The listing builds one solid part. Answer for the finished solid, in the listing's coordinates (mm). Round coordinates to 2 decimals unless told otherwise and drop trailing zeros. Loops run counter-clockwise (first coordinate to the right, second up) from the corner with the lowest first, then second, coordinate; pieces in that order, holes last. Notation, with made-up numbers: M -38,-22.75 L 15,-22.75 A33 cw 15,6.25 Z; hole C 81.25,26.5 d9. An arc over 180 degrees is marked long. Put each result on its own line as item: value. Start each with the question number.
(1) Determine the mould class of faces 1 (the face through (-5, 0, 50)), 2 (the face through (-0.59, -4.46, -0.7)), 3 (the face through (-1.19, -5.37, 32.75)) for opening direction Y: released by +Y, released by -Y, zero draft, split by the parting line, or undercut.
(2) Section D-D, the plane z = -38 is taken. Determine the outline of the cut face in (x, y), then the cut area to 3 significant figures.
(3) Straight lines are drawn through the part: line 1 (Y direction, x = 0, z = 19); line 2 (Y direction, x = 0, z = 7); line 3 (X direction, y = -0.75, z = 23.5). For each, find the intervals that lie inside material, in ascending order.
(4) Section C-C, the plane z = 22.5 is taken. Determine the outline of the cut face in (x, y).
(5) Flat-ended cylindrical pins translate along their axes: P1, Ø5.5, axis at x = 1, y = 0.5, coming from the -Z side; P2, Ø2, axis at x = 1, z = 17.5, coming from the -Y side; P3, Ø4, axis at y = 3, z = 11.5, coming from the +X side; P4, Ø1, axis at y = 4.5, z = 7.5, coming from the -X side. Find the tip coordinate at first contact, or state that the pin passes through.
(6) Section A-A, the plane y = 0 is taken. Determine the outline of the cut face in (x, z), then the cut area to 3 significant figures.
```python
from build123d import *

# Parameters (mm, degrees)
F0_R     = 5
F1_DEPTH = 50
F3_R     = 4.5
F4_DEPTH = 100
F5_R     = 5.5
F5_R_2   = 5
F6_DEPTH = 35


with BuildPart() as f1:
    # F0 (on Top) → F1 (new body)
    with BuildSketch(Plane.XY):
        Circle(F0_R)
    extrude(amount=F1_DEPTH)

    # F2: F1 across face


with BuildPart() as f1_1:
    add(f1.part)
    add(f1.part.mirror(Plane(origin=(0, 0, 0), x_dir=(1, 0, 0), z_dir=(0, 0, -1))))

    # F3 (on face) → F4 (cut)
    with BuildSketch(Plane(origin=(0, 0, -50), x_dir=(1, 0, 0), z_dir=(0, 0, -1))):
        Circle(F3_R)
    extrude(amount=-F4_DEPTH, mode=Mode.SUBTRACT)

    # F5 (on face) → F6 (join)
    with BuildSketch(Plane.XY.offset(50)):
        Circle(F5_R)
        Circle(F5_R_2, mode=Mode.SUBTRACT)
    extrude(amount=-F6_DEPTH)


solid = f1_1.part
```
Recorded:
1. face 1: zero draft
1. face 2: undercut
1. face 3: split by the parting line
2. outline: C 0,0 d10; hole C 0,0 d9
2. area: 14.9 mm²
3. line 1: y = -5.5 to -4.5, 4.5 to 5.5
3. line 2: y = -5 to -4.5, 4.5 to 5
3. line 3: x = -5.45 to -4.44, 4.44 to 5.45
4. outline: C 0,0 d11; hole C 0,0 d9
5. P1: passes through
5. P2: stops at y = -5.5
5. P3: stops at x = 4.9
5. P4: stops at x = -3
6. outline: M -5.5,15 L -5,15 L -5,-50 L -4.5,-50 L -4.5,50 L -5.5,50 Z; M 4.5,-50 L 5,-50 L 5,15 L 5.5,15 L 5.5,50 L 4.5,50 Z
6. area: 135 mm²
